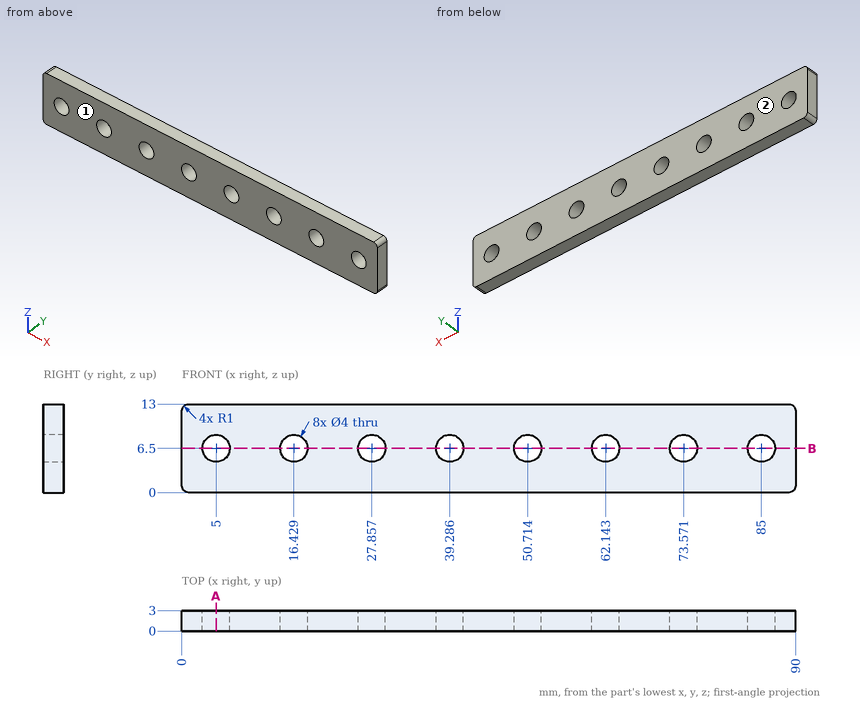
The figure shows three views and two pictorial views of one solid part (mm, origin at its lowest corner). Answer the questions. Round coordinates to 2 decimals unless told otherwise and drop trailing zeros. Loops run counter-clockwise (first coordinate to the right, second up) from the corner with the lowest first, then second, coordinate; pieces in that order, holes last. Notation, with made-up numbers: M -23,-4.5 L -7,-4.5 A10 cw -7,13.5 Z; hole C 82,-25.5 d6. An arc over 180 degrees is marked long. Use CSV: the item, a comma, the result in double quotes.
Q1. Section B-B, the plane z = 6.5 is taken. State how many separate pieces and enclosed holes the cut face has, then the cut area to 3 significant figures.
Determined:
separate pieces,"9"
enclosed holes,"0"
area,"174 mm2"
Q2. Consider L1, parallel to Z at x = 85, y = 1.05; L2, parallel to Z at x = 61.5, y = 1 (1 decimal). Determine where each line is inside the solid, lowest interval first.
Determined:
L1,"0 to 4.5, 8.5 to 13"
L2,"0 to 4.6, 8.4 to 13"
Q3. Section A-A, the plane x = 5 is taken. Determine the outline of the cut face in (y, z).
Determined:
outline,"M 0,0 L 3,0 L 3,4.5 L 0,4.5 Z; M 0,8.5 L 3,8.5 L 3,13 L 0,13 Z"
Q4. The mould has two halves that part along Y. Classify the marked faces 1 and 2: pulls with the +Y half, pulls with the -Y half, needs draft (parallel to the pull), parting line crosses it, or undercut.
Determined:
face 1,"pulls with the -Y half"
face 2,"pulls with the +Y half"
Q5. This flat-tipped pin is pushed along its axis until it touches: pin 1 (2.5 mm diameter, centred on x = 16.43, z = 6.5, fed in from +Y). Where does it stop, or does it pass through?
Determined:
pin 1,"through"
